Can you work these out from the model? Positions are in its coordinate system, mm. Face numbers are marked on the shaded views. A direction names the side the tool comes from. Give positions to 0.01 mm unless a question says otherwise; leave off trailing zeros. Write each loop counter-clockwise with the first axis right and the second up, starting at its lowest first coordinate (ties: lowest second). Pieces come first, ordered by that corner, then holes. Notation, with made-up numbers: (-31.5, -3) -> (22.5, -3) arc R24 ccw to (22.5, 27) -> close; hole circle Ø5 at (13.25, 27.25). An arc over 180 degrees is marked (long way). One line per item, written item: value.
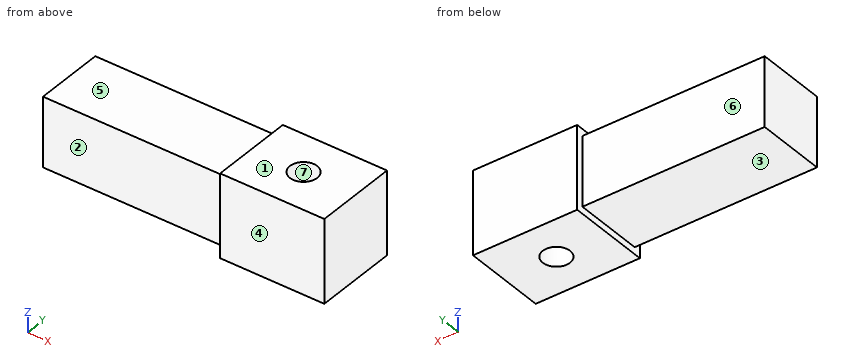
from build123d import *

# Parameters (mm, degrees)
F0_W          = 70
F0_H          = 26.7
F2_DEPTH      = 26.7
F1_W          = 40
F1_H          = 32
F3_DEPTH      = 29.35
F3_DEPTH_BACK = 2.65
F5_D          = 10.5


with BuildPart() as f2:
    # F0 (on Front) → F2 (new body)
    with BuildSketch(Plane.XZ):
        with Locations((-14.08916, 0.31107)):
            Rectangle(F0_W, F0_H)
    extrude(amount=F2_DEPTH)

    # F1 (on Front) → F3 (join, two sides)
    with BuildSketch(Plane.XZ) as f3_sk:
        with Locations((40.91084, 0.31107)):
            Rectangle(F1_W, F1_H)
    extrude(amount=F3_DEPTH)
    extrude(f3_sk.sketch, amount=-F3_DEPTH_BACK)

    # F5 (through all)
    with Locations(Plane.XY.offset(16.31107)):
        with Locations((40.91084, -13.35)):
            Hole(F5_D / 2)


solid = f2.part
1) If we section it at B-B (z = -6): Write out the boundary of the cut face in (x, y).
Answer list:
outline: (-49.09, -26.7) -> (20.91, -26.7) -> (20.91, -29.35) -> (60.91, -29.35) -> (60.91, 2.65) -> (20.91, 2.65) -> (20.91, 0) -> (-49.09, 0) -> close; hole circle Ø10.5 at (40.91, -13.35)
2) If we section it at C-C (x = 37): Write out the boundary of the cut face in (y, z).
Answer list:
outline: (-29.35, -15.69) -> (-16.85, -15.69) -> (-16.85, 16.31) -> (-29.35, 16.31) -> close; (-9.85, -15.69) -> (2.65, -15.69) -> (2.65, 16.31) -> (-9.85, 16.31) -> close
3) We'd pull the mould along Y, two halves only. Please class the marked faces 4, 5, 6 and 7: released by +Y, released by -Y, zero draft, split by the parting line, or undercut.
Answer list:
face 4: released by -Y
face 5: zero draft
face 6: released by +Y
face 7: undercut
4) For the marked faces 1, 2 and 3, which set-ups out of +Z, -Z, +X, -X, +Y, -Y let a thin tool reach every point of the face, with its end or its side?
Answer list:
face 1: +Z, +X, -X, +Y, -Y
face 2: +Z, -Z, -X, -Y
face 3: -Z, -X, +Y, -Y
5) If we section it at A-A (y = -13.35): Write out the boundary of the cut face in (x, z), and give its area (3 significant figures).
Answer list:
outline: (-49.09, -13.04) -> (20.91, -13.04) -> (20.91, -15.69) -> (35.66, -15.69) -> (35.66, 16.31) -> (20.91, 16.31) -> (20.91, 13.66) -> (-49.09, 13.66) -> close; (46.16, -15.69) -> (60.91, -15.69) -> (60.91, 16.31) -> (46.16, 16.31) -> close
area: 2,810 mm^2
6) If we section it at D-D (y = -20.5): Write out the boundary of the cut face in (x, z).
Answer list:
outline: (-49.09, -13.04) -> (20.91, -13.04) -> (20.91, -15.69) -> (60.91, -15.69) -> (60.91, 16.31) -> (20.91, 16.31) -> (20.91, 13.66) -> (-49.09, 13.66) -> close
7) Will these pins go through, and if not, where does the flat tip stop? pin 1 (13.5 mm diameter, centred on x = 40.91, y = -13.35, fed in from -Z); pin 2 (10 mm diameter, centred on x = -25.5, z = -4, fed in from -Y); pin 3 (8 mm diameter, centred on x = -7.5, y = -7, fed in from +Z); pin 4 (2 mm diameter, centred on x = -16, y = -17, fed in from -Z).
Answer list:
pin 1: stops at z = -15.69
pin 2: stops at y = -26.7
pin 3: stops at z = 13.66
pin 4: stops at z = -13.04
8) I need wall thicknesses on L1, parallel to X at y = -13, z = 5; L2, parallel to Y at x = -25, z = -4.5; L3, parallel to Z at x = -3.5, y = -23.5. Which ranges of each line are inside material? Lowest first, please.
Answer list:
L1: x = -49.09 to 35.67, 46.15 to 60.91
L2: y = -26.7 to 0
L3: z = -13.04 to 13.66
